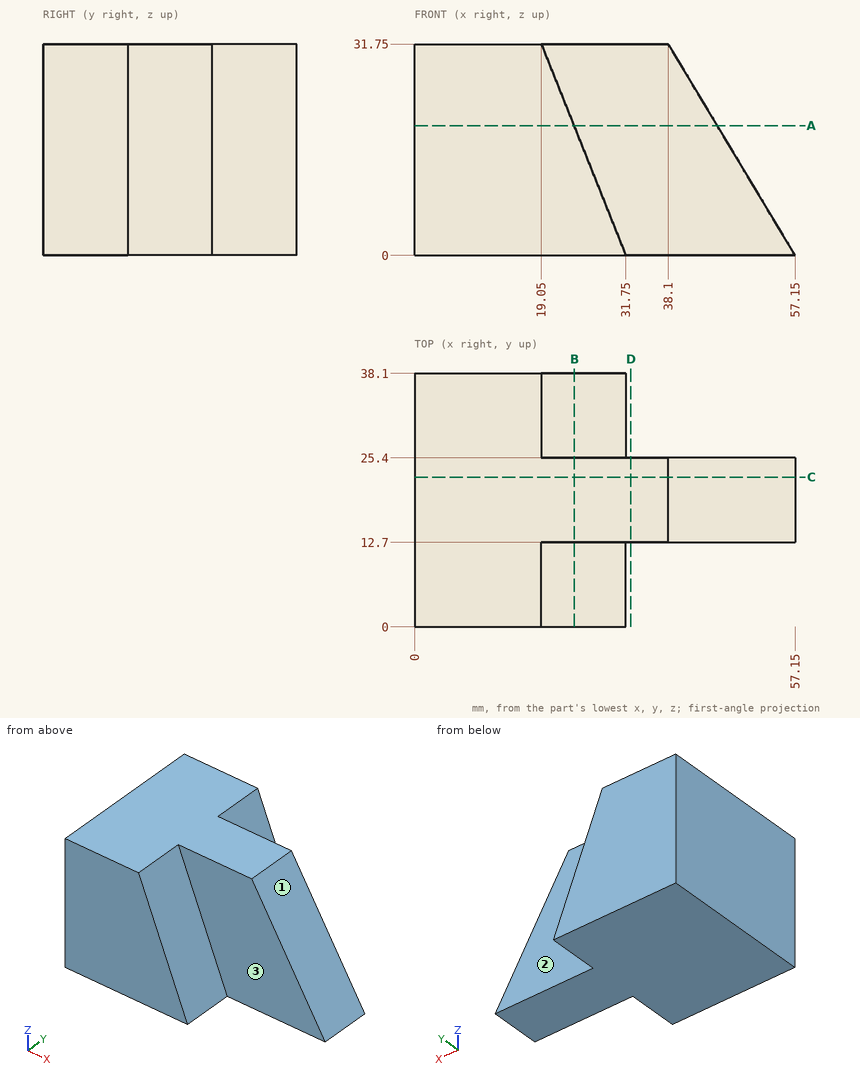
Input: dimensioned drawing with shaded views. Units: mm. Origin: part minimum x, y, z. A direction names the side the tool comes from. Coordinates: 2 decimals unless noted, no trailing zeros. Loops run counter-clockwise (first coordinate to the right, second up) from the corner with the lowest first, then second, coordinate; pieces in that order, holes last.
Q1. Section C-C, the plane y = 22.5. Return the cut outline in (x, z).
Results are:
outline: (0, 0) - (57.15, 0) - (38.1, 31.75) - (0, 31.75) - close
Q2. Line query: line 1 along Y through (x, z) = (26, 18); line 2 along X through (y, z) = (22, 27.5); line 3 along X through (y, z) = (7, 9.5). Output: solid intervals per line, ascending.
Results are:
line 1: y = 12.7 to 25.4
line 2: x = 0 to 40.65
line 3: x = 0 to 27.95
Q3. Section B-B, the plane x = 24. Return the cut outline in (y, z) (3 decimals), and give its area (3 significant figures).
Results are:
outline: (0, 0) - (38.1, 0) - (38.1, 19.375) - (25.4, 19.375) - (25.4, 31.75) - (12.7, 31.75) - (12.7, 19.375) - (0, 19.375) - close
area: 895 mm2
Q4. Section D-D, the plane x = 32.5. Return the cut outline in (y, z), and give its area (3 significant figures).
Results are:
outline: (12.7, 0) - (25.4, 0) - (25.4, 31.75) - (12.7, 31.75) - close
area: 403 mm2
Q5. Set-up query: the marked faces 1, 2 and 3. Return all of +Z, -Z, +X, -X, +Y, -Y with unobstructed straight access to the full face (end or side cutting, diameter ignored); none if empty.
Results are:
face 1: +Z, +X, +Y, -Y
face 2: +Z, +X, +Y
face 3: +Z, +X, -Y
Q6. Section A-A, the plane z = 19.5. Return the cut outline in (x, y).
Results are:
outline: (0, 0) - (23.95, 0) - (23.95, 12.7) - (45.45, 12.7) - (45.45, 25.4) - (23.95, 25.4) - (23.95, 38.1) - (0, 38.1) - close
Q7. Contact query for flat-ended pins moving along their axis: pin 1 (5 mm diameter, centred on y = 6.5, z = 20, fed in from +X); pin 2 (1.5 mm diameter, centred on y = 20.5, z = 4.5, fed in from +X); pin 3 (9.5 mm diameter, centred on x = 41.5, z = 10.5, fed in from -Y); pin 4 (10 mm diameter, centred on x = 16, y = 15, fed in from -Z). Output: stop coordinate, or through.
Results are:
pin 1: stops at x = 24.75
pin 2: stops at x = 54.9
pin 3: stops at y = 12.7
pin 4: stops at z = 0
